CAD build for the part. Positions are in the model's coordinates, mm. Coordinates: 2 decimals unless noted, no trailing zeros. Loops run counter-clockwise (first coordinate to the right, second up) from the corner with the lowest first, then second, coordinate; pieces in that order, holes last. Notation, with made-up numbers: (-30.5, -3) - (4.5, -3) arc R26 ccw to (4.5, 24) - close; hole circle Ø3 at (66.5, -10). An arc over 180 degrees is marked (long way). Put each result on its own line as item: value.
```python
from build123d import *

# Parameters (mm, degrees)
SKETCH1_R           = 1.7272
BOSS_EXTRUDE1_DEPTH = 3.175
FILLET2_R           = 7.62


with BuildPart() as part:
    # Sketch1 → Boss-Extrude1 (new body)
    with BuildSketch(Plane(origin=(0, 0, 0), x_dir=(1, 0, 0), z_dir=(0, 1, 0))):
        with BuildLine():
            Line((-8.4836, 76.2), (-8.4836, 69.332900062))
            ThreePointArc((-8.4836, 69.332900062), (-49.391408666, 49.391408666), (-69.332900062, 8.4836))
            Line((-69.332900062, 8.4836), (-76.2, 8.4836))
            ThreePointArc((-76.2, 8.4836), (-84.6836, 0), (-76.2, -8.4836))
            Line((-76.2, -8.4836), (-69.332900062, -8.4836))
            ThreePointArc((-69.332900062, -8.4836), (-49.391408666, -49.391408666), (-8.4836, -69.332900062))
            Line((-8.4836, -69.332900062), (-8.4836, -76.2))
            ThreePointArc((-8.4836, -76.2), (0, -84.6836), (8.4836, -76.2))
            Line((8.4836, -76.2), (8.4836, -69.332900062))
            ThreePointArc((8.4836, -69.332900062), (49.391408666, -49.391408666), (69.332900062, -8.4836))
            Line((69.332900062, -8.4836), (76.2, -8.4836))
            ThreePointArc((76.2, -8.4836), (84.6836, 0), (76.2, 8.4836))
            Line((76.2, 8.4836), (69.332900062, 8.4836))
            ThreePointArc((69.332900062, 8.4836), (49.391408666, 49.391408666), (8.4836, 69.332900062))
            Line((8.4836, 69.332900062), (8.4836, 76.2))
            ThreePointArc((8.4836, 76.2), (0, 84.6836), (-8.4836, 76.2))
        make_face()
        with Locations(Location((0, 76.2, 0), (0, 0, 270))):
            Circle(SKETCH1_R, mode=Mode.SUBTRACT)
        with Locations(Location((76.2, 0, 0), (0, 0, 270))):
            Circle(SKETCH1_R, mode=Mode.SUBTRACT)
        with Locations(Location((0, -76.2, 0), (0, 0, 270))):
            Circle(SKETCH1_R, mode=Mode.SUBTRACT)
        with Locations(Location((-76.2, 0, 0), (0, 0, 270))):
            Circle(SKETCH1_R, mode=Mode.SUBTRACT)
    extrude(amount=BOSS_EXTRUDE1_DEPTH)

    # Fillet2
    fillet2_edges = [part.edges().sort_by_distance(p)[0] for p in [
        (8.4836, 1.5875, -69.332900062),
        (69.332900062, 1.5875, -8.4836),
        (69.332900062, 1.5875, 8.4836),
        (8.4836, 1.5875, 69.332900062),
        (-8.4836, 1.5875, 69.332900062),
        (-69.332900062, 1.5875, 8.4836),
        (-69.332900062, 1.5875, -8.4836),
        (-8.4836, 1.5875, -69.332900062),
    ]]
    fillet(fillet2_edges, radius=FILLET2_R)


solid = part.part
```
Q1. Slice it at C-C, the plane z = 35.5. Give the cut face in (x, y) (3 decimals), then the cut area to 3 significant figures.
Determined:
outline: (-60.156, 0) - (60.156, 0) - (60.156, 3.175) - (-60.156, 3.175) - close
area: 382 mm2
Q2. Slice it at A-A, the plane y = 1.15. Give the cut face in (x, z).
Determined:
outline: (-76.2, -8.48) - (-75.78, -8.48) arc R7.62 cw to (-68.32, -14.52) arc R69.85 ccw to (-14.52, -68.32) arc R7.62 cw to (-8.48, -75.78) - (-8.48, -76.2) arc R8.48 ccw to (8.48, -76.2) - (8.48, -75.78) arc R7.62 cw to (14.52, -68.32) arc R69.85 ccw to (68.32, -14.52) arc R7.62 cw to (75.78, -8.48) - (76.2, -8.48) arc R8.48 ccw to (76.2, 8.48) - (75.78, 8.48) arc R7.62 cw to (68.32, 14.52) arc R69.85 ccw to (14.52, 68.32) arc R7.62 cw to (8.48, 75.78) - (8.48, 76.2) arc R8.48 ccw to (-8.48, 76.2) - (-8.48, 75.78) arc R7.62 cw to (-14.52, 68.32) arc R69.85 ccw to (-68.32, 14.52) arc R7.62 cw to (-75.78, 8.48) - (-76.2, 8.48) arc R8.48 ccw to start; hole circle Ø3.45 at (-76.2, 0); hole circle Ø3.45 at (0, -76.2); hole circle Ø3.45 at (0, 76.2); hole circle Ø3.45 at (76.2, 0)
Q3. Slice it at B-B, the plane x = 11. Give the cut face in (y, z) (3 decimals).
Determined:
outline: (0, -70.119) - (3.175, -70.119) - (3.175, 70.119) - (0, 70.119) - close
Q4. Wall check: L1, parallel to X at y = 1.8, z = 0; L2, parallel to X at y = 1.9, z = 76.2. Give the ranges that are in metal, low to high. Write a range as from..to.
Determined:
L1: -84.68..-77.93, -74.47..74.47, 77.93..84.68
L2: -8.48..-1.73, 1.73..8.48
Q5. Pin check, flat tips, straight feed: pin 1 Ø4 at (x, z) = (76.2, 0) entering from -Y; pin 2 Ø1 at (x, y) = (41.5, 1.5) entering from -Z; pin 3 Ø0.5 at (y, z) = (1.5, 76) entering from -X; pin 4 Ø0.5 at (x, y) = (-76, 1.5) entering from +Z. Stop position of each tip, or through.
Determined:
pin 1: y = 0
pin 2: z = -56.55
pin 3: x = -8.48
pin 4: z = 8.48
